The listing builds one solid part. Answer for the finished solid, in the listing's coordinates (mm). A direction names the side the tool comes from. Coordinates: 2 decimals unless noted, no trailing zeros. Write each loop counter-clockwise with the first axis right and the second up, starting at its lowest first coordinate (ties: lowest second). Pieces come first, ordered by that corner, then holes. Notation, with made-up numbers: M 51.25,52.5 L 67.25,52.5 A25 cw 67.25,70.5 Z; hole C 65,52 d9. An arc over 180 degrees is marked long. Answer as a JSON object with one key per item and string values. Group by question number.
from build123d import *

# Parameters (mm, degrees)
BOSS_EXTRUDE1_DEPTH = 16
CUT_EXTRUDE1_REACH  = 10.836
SKETCH2_R           = 1.6


with BuildPart() as part:
    # Sketch1 → Boss-Extrude1 (new body)
    with BuildSketch(Plane(origin=(0, 0, 0), x_dir=(1, 0, 0), z_dir=(0, 1, 0))):
        with BuildLine():
            Line((-1.728929985, 4.409979173), (-5.295587342, 4.409979173))
            ThreePointArc((-5.295587342, 4.409979173), (-4.887048333, 2.349132427), (-4.465862239, 0.290833199))
            ThreePointArc((-4.465862239, 0.290833199), (-2.551857479, -2.856477369), (0.919071585, -4.090020827))
            Line((0.919071585, -4.090020827), (4.376171699, -4.090020827))
            Line((4.376171699, -4.090020827), (4.376171699, -0.590020827))
            Line((4.376171699, -0.590020827), (-1.728929985, 4.409979173))
        make_face()
        with BuildLine():
            Line((-1.728929985, 3.409979173), (3.376171699, -0.590020827))
            Line((3.376171699, -0.590020827), (3.376171699, -3.090020827))
            Line((3.376171699, -3.090020827), (0.919071585, -3.090020827))
            ThreePointArc((0.919071585, -3.090020827), (-1.920779468, -2.080757998), (-3.486783362, 0.494314286))
            ThreePointArc((-3.486783362, 0.494314286), (-3.786316073, 1.951500554), (-4.079491423, 3.409979173))
            Line((-4.079491423, 3.409979173), (-1.728929985, 3.409979173))
        make_face(mode=Mode.SUBTRACT)
    extrude(amount=BOSS_EXTRUDE1_DEPTH)

    # Cut-Extrude1: up to this face of the body (flat: up to its plane)
    cut_extrude1_end = Plane(part.part.faces().sort_by_distance((0.823620857, 8, -1.409979173))[0])
    # Sketch2 → Cut-Extrude1 (cut, up to the picked face)
    with BuildSketch(Plane(origin=(1.467645419, 0, -1.792024904), x_dir=(-0.773651844, 0, -0.633610941), z_dir=(0.633610941, 0, -0.773651844)), mode=Mode.PRIVATE) as cut_extrude1_sk1:
        with Locations((0.093080992, 8)):
            Circle(SKETCH2_R)
    cut_extrude1_tool1 = split(extrude(cut_extrude1_sk1.sketch, amount=-CUT_EXTRUDE1_REACH, mode=Mode.PRIVATE), bisect_by=cut_extrude1_end, keep=Keep.BOTH, mode=Mode.PRIVATE)
    add(cut_extrude1_tool1.solids().sort_by_distance((1.395633, 8, -1.851002))[0], mode=Mode.SUBTRACT)


solid = part.part
Item 1: A tool of negligible diameter and unlimited length cuts with its end or side. For faces 4 (the face through (3, 8, 4.09)), 5 (the face through (-1.9, 7.9, 2.1)), from which of +Z, -Z, +X, -X, +Y, -Y can it reach the whole face along a straight path? Write none if from no direction.
Item 2: A cutting plane is placed at B-B, the plane x = -2.25. Write down the section's boundary in (y, z), and give its area (3 significant figures).
Item 3: A cutting plane is placed at C-C, the plane z = 2.5. Write down the section's boundary in (x, y).
Item 4: For a pull along X with two mould halves and no side action, classify faces 1 (the face through (-3, 8, -4.41)), 2 (the face through (0.01, 7.888, -2.986)), 3 (the face through (0.788, 6.11, -1.438)) as +X half, -X half, draft (parallel to the pull), parting line (faces both ways), or undercut.
Item 5: Consider L1, parallel to Z at x = -2.5, y = 5.25; L2, parallel to Z at x = -2, y = 12.5; L3, parallel to X at y = 12.75, z = 0. Determine where each line is inside the solid, lowest interval first. Write a range as from..to.
Item 6: Flat-ended cylindrical pins translate along their axes: pin 1 Ø4 at (y, z) = (5.5, -1.5) entering from +X; pin 2 Ø0.8 at (y, z) = (7, 1.5) entering from -X; pin 3 Ø1.9 at (x, y) = (-3.5, 10.5) entering from +Z; pin 4 Ø1.5 at (x, z) = (-0.5, -0.5) entering from -Y. Find the tip coordinate at first contact, or state that the pin passes through.
Item 7: A cutting plane is placed at A-A, the plane y = 11. Write down the section's boundary in (x, z).
Item 8: A cutting plane is placed at D-D, the plane z = -1. State how many separate pieces and enclosed holes the cut face has, and give its area (3 significant figures).
Answer:
{
 "1": {"face 4": "+Z, +X, -X, +Y, -Y", "face 5": "+Y, -Y"},
 "2": {"outline": "M 0,-4.41 L 16,-4.41 L 16,-3.41 L 0,-3.41 Z; M 0,1.78 L 16,1.78 L 16,3.09 L 0,3.09 Z", "area": "36.8 mm2"},
 "3": {"outline": "M -2.95,0 L -1.31,0 L -1.31,16 L -2.95,16 Z; M 3.38,0 L 4.38,0 L 4.38,16 L 3.38,16 Z"},
 "4": {"face 1": "draft", "face 2": "+X half", "face 3": "undercut"},
 "5": {"L1": "-4.41..-3.41, 1.52..2.9", "L2": "-4.41..-3.41, 2.01..3.25", "L3": "-4.4..-3.35, 2.62..3.66"},
 "6": {"pin 1": "x = 4.27", "pin 2": "x = -3.97", "pin 3": "z = 2.86", "pin 4": "through"},
 "7": {"outline": "M -5.3,-4.41 L -1.73,-4.41 L 4.38,0.59 L 4.38,4.09 L 0.92,4.09 A5.5 ccw -4.47,-0.29 A342.14 ccw Z; hole M -4.08,-3.41 L -1.73,-3.41 L 3.38,0.59 L 3.38,3.09 L 0.92,3.09 A4.5 ccw -3.49,-0.49 A341.14 ccw Z"},
 "8": {"separate pieces": "3", "enclosed holes": "0", "area": "31.0 mm2"}
}
